```python
from build123d import *

# Parameters (mm, degrees)
SKETCH1_W            = 20
SKETCH1_H            = 7
SKETCH1_R            = 1.15
BOSS_EXTRUDE1_DEPTH  = 2
BOSS_EXTRUDE11_DEPTH = 10
BOSS_EXTRUDE12_DEPTH = 1
SKETCH8_W            = 10
SKETCH8_H            = 1
BOSS_EXTRUDE13_DEPTH = 5


with BuildPart() as part:
    # Sketch1 → Boss-Extrude1 (new body)
    with BuildSketch(Plane.XY):
        with Locations((10, 3.5)):
            Rectangle(SKETCH1_W, SKETCH1_H)
        with Locations((1.75, 3.5)):
            Circle(SKETCH1_R, mode=Mode.SUBTRACT)
        with Locations((18.25, 3.5)):
            Circle(SKETCH1_R, mode=Mode.SUBTRACT)
        with BuildLine():
            Line((7, 4.75), (13, 4.75))
            ThreePointArc((13, 4.75), (14.25, 3.5), (13, 2.25))
            Line((13, 2.25), (7, 2.25))
            ThreePointArc((7, 2.25), (5.75, 3.5), (7, 4.75))
        make_face(mode=Mode.SUBTRACT)
    extrude(amount=BOSS_EXTRUDE1_DEPTH)

    # Sketch6 → Boss-Extrude11 (add)
    with BuildSketch(Plane.XY.offset(2)):
        with BuildLine():
            Line((7.233144363, 5.202021214), (12.654721, 5.20752793))
            ThreePointArc((12.654721, 5.20752793), (14.690102928, 3.922399472), (13.498649888, 1.830803334))
            Line((13.498649888, 1.830803334), (15, 1.830803334))
            Line((15, 1.830803334), (15, 0.830803334))
            Line((15, 0.830803334), (5, 0.830803334))
            Line((5, 0.830803334), (5, 1.830803334))
            Line((5, 1.830803334), (6.593779621, 1.830803334))
            ThreePointArc((6.593779621, 1.830803334), (5.312171121, 3.820103391), (7.233144363, 5.202021214))
        make_face()
        with BuildLine():
            Line((7, 4.77), (13, 4.77))
            ThreePointArc((13, 4.77), (14.27, 3.5), (13, 2.23))
            Line((13, 2.23), (7, 2.23))
            ThreePointArc((7, 2.23), (5.73, 3.5), (7, 4.77))
        make_face(mode=Mode.SUBTRACT)
    extrude(amount=BOSS_EXTRUDE11_DEPTH)

    # Sketch7 → Boss-Extrude12 (add)
    with BuildSketch(Plane.XY.offset(12)):
        with BuildLine():
            Line((7, 5.233060679), (13, 5.233060679))
            ThreePointArc((13, 5.233060679), (14.733060679, 3.5), (13, 1.766939321))
            Line((13, 1.766939321), (7, 1.766939321))
            ThreePointArc((7, 1.766939321), (5.266939321, 3.5), (7, 5.233060679))
        make_face()
    extrude(amount=-BOSS_EXTRUDE12_DEPTH)

    # Sketch8 → Boss-Extrude13 (add)
    with BuildSketch(Plane.XY.offset(12)):
        with Locations((10, 1.330803334)):
            Rectangle(SKETCH8_W, SKETCH8_H)
    extrude(amount=BOSS_EXTRUDE13_DEPTH)


solid = part.part
```
Part model, mm, in its own coordinate system. A direction names the side the tool comes from. Round coordinates to 2 decimals unless told otherwise and drop trailing zeros. Loops run counter-clockwise (first coordinate to the right, second up) from the corner with the lowest first, then second, coordinate; pieces in that order, holes last.
Item 1: Cut at A-A, the plane x = 18.25. Give the cut face in (y, z), then the cut area to 3 significant figures.
Item 2: 3-axis set-ups, long thin cutter, end or side, ignore diameter. For faces 1 (the face through (5.73, 3.47, 6.44)), 2 (the face through (5.75, 3.47, 0.99)), 3 (the face through (10, 0.831, 9)): which of +Z, -Z, +X, -X, +Y, -Y reach the whole face in a straight line?
Item 3: Cut at B-B, the plane y = 3.5. State how many separate pieces and enclosed holes the cut face has, then the cut area to 3 significant figures.
Item 4: Drop flat-ended pins along their axis: P1, Ø2.5, axis at x = 18.25, y = 3.5, coming from the -Z side; P2, Ø3, axis at y = 6, z = 13, coming from the +X side; P3, Ø0.8, axis at y = 1.5, z = 10.5, coming from the +X side; P4, Ø2, axis at x = 10, y = 4.5, coming from the +Z side. Give the stop position or say it passes through.
Item 5: Mould opens along X. For faces 4 (the face through (10, 2, 0)), 5 (the face through (5, 1, 9)), 6 (the face through (10, 2.25, 1)) say: +X half, -X half, draft (parallel to the pull), parting line (faces both ways), or undercut.
Item 6: Cut at C-C, the plane z = 5.25. Give the cut face in (x, y), then the cut area to 3 significant figures.
Item 7: Drill centre lines: line 1 (Y direction, x = 9.5, z = 8.5); line 2 (Y direction, x = 18.25, z = 1); line 3 (Y direction, x = 12.5, z = 11.5). Where is each one in solid material? Low to high.
A:
1. outline: (0, 0) - (2.35, 0) - (2.35, 2) - (0, 2) - close; (4.65, 0) - (7, 0) - (7, 2) - (4.65, 2) - close
1. area: 9.40 mm2
2. face 1: none
2. face 2: -Z
2. face 3: +Z, +X, -X, -Y
3. separate pieces: 3
3. enclosed holes: 0
3. area: 31.6 mm2
4. P1: stops at z = 0
4. P2: stops at x = 14.06
4. P3: stops at x = 15
4. P4: stops at z = 12
5. face 4: draft
5. face 5: -X half
5. face 6: undercut
6. outline: (5, 0.83) - (15, 0.83) - (15, 1.83) - (13.5, 1.83) arc R1.74 ccw to (12.65, 5.21) - (7.23, 5.2) arc R1.72 ccw to (6.59, 1.83) - (5, 1.83) - close; hole (7, 2.23) - (13, 2.23) arc R1.27 ccw to (13, 4.77) - (7, 4.77) arc R1.27 ccw to start
6. area: 19.3 mm2
7. line 1: y = 0.83 to 2.23, 4.77 to 5.2
7. line 2: y = 0 to 2.35, 4.65 to 7
7. line 3: y = 0.83 to 5.23
